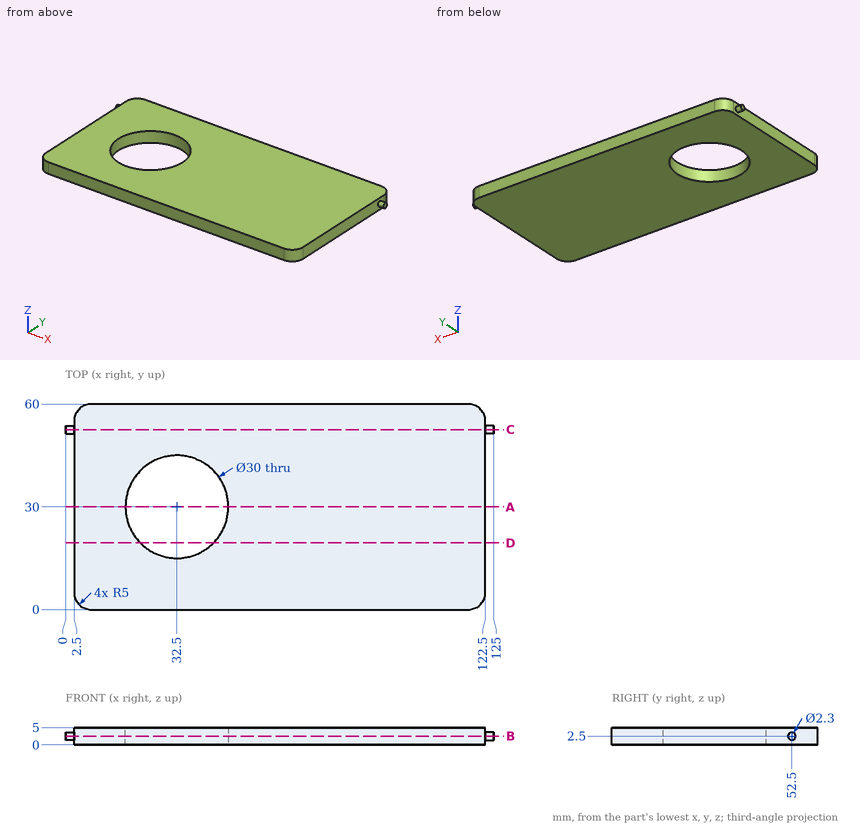
Part print with two shaded views. Sizes in mm from the minimum x, y, z corner. Give positions to 0.01 mm unless a question says otherwise; leave off trailing zeros. Order: outer loops, then holes, each group sorted by start corner. A loop starts at its lowest first (then second) coordinate and runs counter-clockwise, first axis right, second up. Notation, with made-up numbers: (62, -21.5) - (111, -21.5) arc R16 cw to (111, 1.5) - close; hole circle Ø11 at (31.5, 43.5). An arc over 180 degrees is marked (long way). Write each question's results on one line, items separated by ' | '.
1. Saw through at D-D on y = 19.5. List the corners of the cut face in (x, z).
Calculated:
outline: (2.5, 0) - (21.79, 0) - (21.79, 5) - (2.5, 5) - close; (43.21, 0) - (122.5, 0) - (122.5, 5) - (43.21, 5) - close
2. Probe L1, parallel to Y at x = 32.5, z = 1.9; L2, parallel to X at y = 40.5, z = 2.95; L3, parallel to X at y = 11, z = 3.3. List the from-to ranges inside material, lowest first. Write a range as from..to.
Calculated:
L1: y = 0..15, 45..60 | L2: x = 2.5..21.79, 43.21..122.5 | L3: x = 2.5..122.5
3. Pin check, flat tip, straight feed: pin 1 (1.5 mm diameter, centred on y = 34, z = 2, fed in from -X). Stop position of the tip, or through.
Calculated:
pin 1: stops at x = 2.5
4. Saw through at C-C on y = 52.5. List the corners of the cut face in (x, z), and give its area (4 significant figures).
Calculated:
outline: (0, 1.35) - (2.5, 1.35) - (2.5, 0) - (122.5, 0) - (122.5, 1.35) - (125, 1.35) - (125, 3.65) - (122.5, 3.65) - (122.5, 5) - (2.5, 5) - (2.5, 3.65) - (0, 3.65) - close | area: 611.5 mm2
5. Saw through at B-B on z = 2.5. List the corners of the cut face in (x, y), and give its area (3 significant figures).
Calculated:
outline: (0, 51.35) - (2.5, 51.35) - (2.5, 5) arc R5 ccw to (7.5, 0) - (117.5, 0) arc R5 ccw to (122.5, 5) - (122.5, 51.35) - (125, 51.35) - (125, 53.65) - (122.5, 53.65) - (122.5, 55) arc R5 ccw to (117.5, 60) - (7.5, 60) arc R5 ccw to (2.5, 55) - (2.5, 53.65) - (0, 53.65) - close; hole circle Ø30 at (32.5, 30) | area: 6,480 mm2
6. Saw through at A-A on y = 30. List the corners of the cut face in (x, z).
Calculated:
outline: (2.5, 0) - (17.5, 0) - (17.5, 5) - (2.5, 5) - close; (47.5, 0) - (122.5, 0) - (122.5, 5) - (47.5, 5) - close
